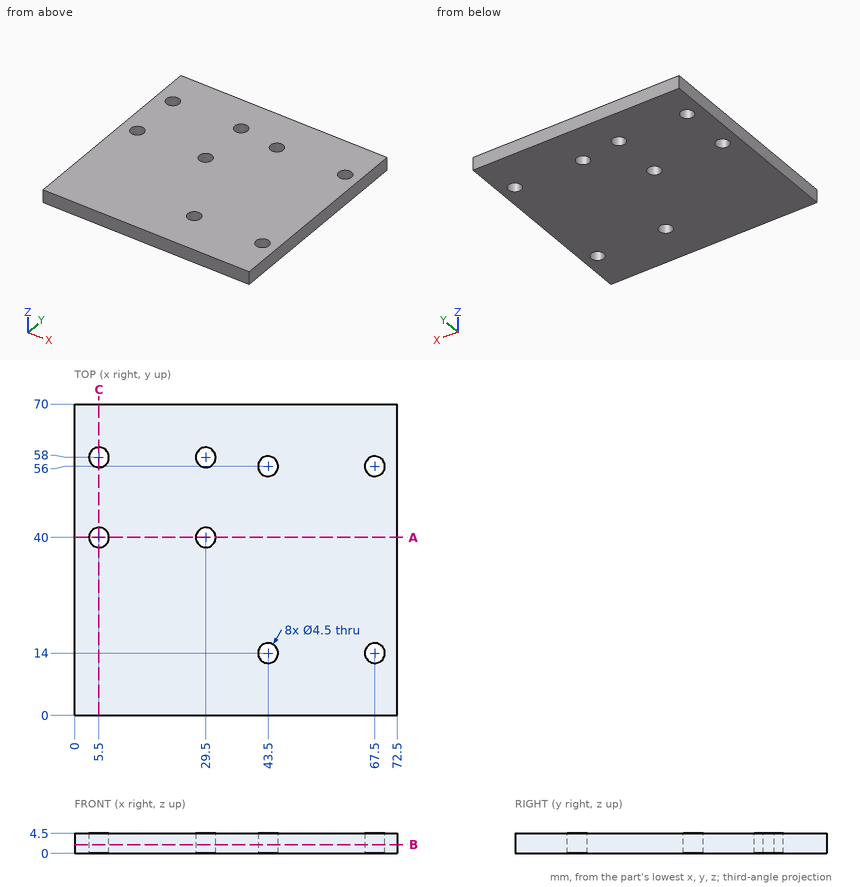
Geometry: see drawing. Coordinates: mm, zero at the bounding-box minimum. Give positions to 0.01 mm unless a question says otherwise; leave off trailing zeros. Order: outer loops, then holes, each group sorted by start corner. A loop starts at its lowest first (then second) coordinate and runs counter-clockwise, first axis right, second up.
Q1. Section A-A on y = 40. Output: boundary loops of the cut face in (x, z).
Checked values:
outline: (0, 0) - (3.25, 0) - (3.25, 4.5) - (0, 4.5) - close; (7.75, 0) - (27.25, 0) - (27.25, 4.5) - (7.75, 4.5) - close; (31.75, 0) - (72.5, 0) - (72.5, 4.5) - (31.75, 4.5) - close
Q2. Section C-C on x = 5.5. Output: boundary loops of the cut face in (y, z).
Checked values:
outline: (0, 0) - (37.75, 0) - (37.75, 4.5) - (0, 4.5) - close; (42.25, 0) - (55.75, 0) - (55.75, 4.5) - (42.25, 4.5) - close; (60.25, 0) - (70, 0) - (70, 4.5) - (60.25, 4.5) - close
Q3. Section B-B on z = 2. State how many separate pieces and enclosed holes the cut face has, and give its area (3 significant figures).
Checked values:
separate pieces: 1
enclosed holes: 8
area: 4,950 mm2
Q4. Contact query for flat-ended pins moving along their axis: pin 1 Ø3.5 at (x, y) = (43.5, 56) entering from -Z; pin 2 Ø5 at (x, y) = (29.5, 40) entering from +Z. Output: stop coordinate, or through.
Checked values:
pin 1: passes through
pin 2: stops at z = 4.5
Q5. Ray query, probe 1 along X at (y, z) = (14, 1.15); probe 2 along Y at (x, z) = (67.5, 1.65); probe 3 along X at (y, z) = (40, 1.05). Return the intervals inside material, ascending.
Checked values:
probe 1: x = 0 to 41.25, 45.75 to 65.25, 69.75 to 72.5
probe 2: y = 0 to 11.75, 16.25 to 53.75, 58.25 to 70
probe 3: x = 0 to 3.25, 7.75 to 27.25, 31.75 to 72.5
